```python
from build123d import *

# Parameters (mm, degrees)
SKETCH_1_R          = 17
SKETCH_1_R_2        = 2
SKETCH_1_R_3        = 8
EXTRUDE_1_DEPTH     = 5.5
EXTRUDE_START       = 5.5
SKETCH_1_3_R        = 2
SKETCH_1_3_R_2      = 3
SKETCH_1_3_R_3      = 8
EXTRUDE_2_DEPTH     = 5
SKETCH_2_R          = 3.25
CUT_EXTRUDE_4_DEPTH = 6
SKETCH_3_W          = 8
SKETCH_3_H          = 2
CUT_EXTRUDE_5_DEPTH = 3


with BuildPart() as part:
    # 스케치1 → 보스-돌출1 (new body)
    with BuildSketch(Plane(origin=(0, 0, 0), x_dir=(1, 0, 0), z_dir=(0, 1, 0))):
        with Locations(Location((0, 0, 0), (0, 0, 270))):
            Circle(SKETCH_1_R)
        with Locations(Location((0, 12, 0), (0, 0, 270))):
            Circle(SKETCH_1_R_2, mode=Mode.SUBTRACT)
        with Locations(Location((10.392304845, 6, 0), (0, 0, 270))):
            Circle(SKETCH_1_R_2, mode=Mode.SUBTRACT)
        with Locations(Location((10.392304845, -6, 0), (0, 0, 270))):
            Circle(SKETCH_1_R_2, mode=Mode.SUBTRACT)
        with Locations(Location((0, -12, 0), (0, 0, 270))):
            Circle(SKETCH_1_R_2, mode=Mode.SUBTRACT)
        with Locations(Location((-10.392304845, -6, 0), (0, 0, 270))):
            Circle(SKETCH_1_R_2, mode=Mode.SUBTRACT)
        with Locations(Location((-10.392304845, 6, 0), (0, 0, 270))):
            Circle(SKETCH_1_R_2, mode=Mode.SUBTRACT)
        with Locations(Location((0, 0, 0), (0, 0, 270))):
            Circle(SKETCH_1_R_3, mode=Mode.SUBTRACT)
    extrude(amount=EXTRUDE_1_DEPTH)

    # 스케치1<3> → 보스-돌출2 (add)
    with BuildSketch(Plane(origin=(0, 0, 0), x_dir=(1, 0, 0), z_dir=(0, 1, 0)).offset(EXTRUDE_START)):
        with BuildLine():
            Line((36.714285714, 4.696937778), (5.828571429, 15.969588445))
            ThreePointArc((5.828571429, 15.969588445), (-17, 0), (5.828571429, -15.969588445))
            Line((5.828571429, -15.969588445), (36.714285714, -4.696937778))
            ThreePointArc((36.714285714, -4.696937778), (40, 0), (36.714285714, 4.696937778))
        make_face()
        with Locations(Location((10.392304845, -6, 0), (0, 0, 270))):
            Circle(SKETCH_1_3_R, mode=Mode.SUBTRACT)
        with Locations(Location((0, -12, 0), (0, 0, 270))):
            Circle(SKETCH_1_3_R, mode=Mode.SUBTRACT)
        with Locations(Location((-10.392304845, -6, 0), (0, 0, 270))):
            Circle(SKETCH_1_3_R, mode=Mode.SUBTRACT)
        with Locations(Location((-10.392304845, 6, 0), (0, 0, 270))):
            Circle(SKETCH_1_3_R, mode=Mode.SUBTRACT)
        with Locations(Location((0, 12, 0), (0, 0, 270))):
            Circle(SKETCH_1_3_R, mode=Mode.SUBTRACT)
        with Locations(Location((10.392304845, 6, 0), (0, 0, 270))):
            Circle(SKETCH_1_3_R, mode=Mode.SUBTRACT)
        with Locations(Location((35, 0, 0), (0, 0, 270))):
            Circle(SKETCH_1_3_R_2, mode=Mode.SUBTRACT)
        with Locations(Location((0, 0, 0), (0, 0, 270))):
            Circle(SKETCH_1_3_R_3, mode=Mode.SUBTRACT)
    extrude(amount=EXTRUDE_2_DEPTH)

    # 스케치2 → 컷-돌출4 (cut)
    with BuildSketch(Plane(origin=(0, 10.5, 0), x_dir=(1, 0, 0), z_dir=(0, 1, 0))):
        with Locations(Location((0, 12, 0), (0, 0, 270))):
            Circle(SKETCH_2_R)
        with Locations(Location((10.392304845, 6, 0), (0, 0, 270))):
            Circle(SKETCH_2_R)
        with Locations(Location((10.392304845, -6, 0), (0, 0, 270))):
            Circle(SKETCH_2_R)
        with Locations(Location((0, -12, 0), (0, 0, 270))):
            Circle(SKETCH_2_R)
        with Locations(Location((-10.392304845, -6, 0), (0, 0, 270))):
            Circle(SKETCH_2_R)
        with Locations(Location((-10.392304845, 6, 0), (0, 0, 270))):
            Circle(SKETCH_2_R)
    extrude(amount=-CUT_EXTRUDE_4_DEPTH, mode=Mode.SUBTRACT)

    # 스케치3 → 컷-돌출5 (cut)
    with BuildSketch(Plane(origin=(0, 10.5, 0), x_dir=(1, 0, 0), z_dir=(0, 1, 0))):
        with Locations((35, 0)):
            Rectangle(SKETCH_3_W, SKETCH_3_H)
    extrude(amount=-CUT_EXTRUDE_5_DEPTH, mode=Mode.SUBTRACT)


solid = part.part
```
Verification items for the finished model (mm, model axes). A direction names the side the tool comes from. Coordinates: 2 decimals unless noted, no trailing zeros. Write each loop counter-clockwise with the first axis right and the second up, starting at its lowest first coordinate (ties: lowest second). Pieces come first, ordered by that corner, then holes. Notation, with made-up numbers: (14.5, 37) - (59.5, 37) arc R23 ccw to (59.5, 46) - close; hole circle Ø1 at (4, 53). An arc over 180 degrees is marked (long way). Write item = value, one per line.
Q1. Mould release check, pull along Z, two halves, no side actions. Record for faces 1 (the face through (40, 8, 0)), 2 (the face through (38, 9, 1)), 3 (the face through (11, 10.5, 0)): released by +Z, released by -Z, zero draft, split by the parting line, or undercut.
Answer:
face_1 = split by the parting line
face_2 = undercut
face_3 = zero draft
Q2. Cross-section at D-D (z = -12). Enter the section's corners in (x, y).
Answer:
outline = (-12.04, 0) - (-2, 0) - (-2, 4.5) - (-3.25, 4.5) - (-3.25, 10.5) - (-12.04, 10.5) - close; (2, 0) - (12.04, 0) - (12.04, 5.5) - (16.7, 5.5) - (16.7, 10.5) - (3.25, 10.5) - (3.25, 4.5) - (2, 4.5) - close
Q3. Cross-section at A-A (z = 0). Enter the section's corners in (x, y), plus the area to 3 significant figures.
Answer:
outline = (-17, 0) - (-8, 0) - (-8, 10.5) - (-17, 10.5) - close; (8, 0) - (17, 0) - (17, 5.5) - (32, 5.5) - (32, 7.5) - (31, 7.5) - (31, 10.5) - (8, 10.5) - close; (38, 5.5) - (40, 5.5) - (40, 10.5) - (39, 10.5) - (39, 7.5) - (38, 7.5) - close
area = 268 mm²
Q4. Cross-section at B-B (x = 0). Enter the section's corners in (y, z), plus the area to 3 significant figures.
Answer:
outline = (0, -17) - (10.5, -17) - (10.5, -15.25) - (4.5, -15.25) - (4.5, -14) - (0, -14) - close; (0, -10) - (4.5, -10) - (4.5, -8.75) - (10.5, -8.75) - (10.5, -8) - (0, -8) - close; (0, 8) - (10.5, 8) - (10.5, 8.75) - (4.5, 8.75) - (4.5, 10) - (0, 10) - close; (0, 14) - (4.5, 14) - (4.5, 15.25) - (10.5, 15.25) - (10.5, 17) - (0, 17) - close
area = 75.0 mm²
Q5. Go/stop test with flat-tipped pins: pin 1 Ø1.3 at (x, y) = (38, 9) entering from -Z; pin 2 Ø3 at (x, y) = (-7, 8.5) entering from -Z; pin 3 Ø4.5 at (x, z) = (-10.39, -6) entering from +Y. Record where each tip stops, or that it passes through.
Answer:
pin_1 = -4.41
pin_2 = -16.09
pin_3 = 4.5
Q6. Cross-section at C-C (y = 9.75). Give the number of separate pieces and of enclosed holes in the cut face, plus the area to 3 significant figures.
Answer:
separate_pieces = 1
enclosed_holes = 8
area = 876 mm²
Q7. Access from +Z, -Z, +X, -X, +Y, -Y to the whole of each face (thin tool, end or side, straight path). Record for faces 4 (the face through (4, 0, 7.3)), 5 (the face through (-1, 4.5, 14)).
Answer:
face_4 = +Z, -Z, +X, -X, -Y
face_5 = +Y
Q8. Material ranges on L1, parallel to Z at x = 3, y = 8; L2, parallel to X at y = 3.5, z = 0; L3, parallel to X at y = 6, z = -2, recorded low to high. Write a range as from..to.
Answer:
L1 = -16.73..-13.25, -10.75..-7.42, 7.42..10.75, 13.25..16.73
L2 = -17..-8, 8..17
L3 = -16.88..-7.75, 7.75..32.76, 37.24..39.58
